Part model, mm, in its own coordinate system. A direction names the side the tool comes from. Give positions to 0.01 mm unless a question says otherwise; leave off trailing zeros. Write each loop counter-clockwise with the first axis right and the second up, starting at its lowest first coordinate (ties: lowest second). Pieces come first, ordered by that corner, then holes.
Autodesk Fusion 360 part; units mm, degrees
sketch "Sketch1" plane through (0, 0, 0) normal (0, 0, 1) x (1, 0, 0)
  line L0 (0, 0) -> (-180, 0)
  line L1 (-180, 0) -> (-180, 105)
  line L2 (-180, 105) -> (0, 105)
  line L3 (0, 105) -> (0, 0)
  dimension "d1" = 180
  dimension "d2" = 105
extrude "Extrude1" add sketch "Sketch1" along normal blind 15
sketch "Sketch2" plane through (0, 0, 15) normal (0, 0, 1) x (-1, 0, 0)
  line L0 (0, -105) -> (180, -105)
  line L1 (180, -105) -> (180, 0)
  line L2 (180, 0) -> (0, 0)
  line L3 (0, 0) -> (0, -105)
  line L4 (90, 0) -> (73, 0)
  line L5 (90, 0) -> (107, 0)
  line L6 (107, 0) -> (107, -12)
  line L7 (107, -12) -> (104, -12)
  line L8 (104, -12) -> (104, -3)
  line L9 (73, 0) -> (73, -12)
  line L10 (73, -12) -> (76, -12)
  line L11 (76, -12) -> (76, -3)
  line L12 (76, -3) -> (104, -3)
  dimension "d6" = 17
  dimension "d7" = 17
  dimension "d14" = 3
  dimension "d15" = 9
  dimension "d26" = 12
  dimension "d27" = 3
extrude "Extrude3" add sketch "Sketch2" along normal blind 115 contours L2 L4 L5 L6 L7 L8 L9 L10 L11 L12
sketch "Sketch4" plane through (0, 0, 130) normal (0, 0, 1) x (-1, 0, 0)
  line L0 (107, 0) -> (73, 0)
  line L1 (104, -3) -> (104, -12)
  line L2 (104, -12) -> (107, -12)
  line L3 (107, -12) -> (107, 0)
  line L4 (73, -12) -> (76, -12)
  line L5 (76, -12) -> (76, -3)
  line L6 (73, 0) -> (73, -12)
  line L7 (76, -3) -> (104, -3)
sketch "Sketch5" plane through (0, 0, 130) normal (0, 0, 1) x (-1, 0, 0)
  line L0 (76, -3) -> (104, -3)
  line L1 (104, -3) -> (104, -12)
  line L2 (104, -12) -> (76, -12)
  line L3 (76, -12) -> (76, -3)
  line L4 (76, -3) -> (104, -12)
  line L5 (76, -12) -> (104, -3)
  circle A0 centre (90, -7.5) radius 2
  dimension "d28" = 4
extrude "Extrude4" add sketch "Sketch5" against normal blind 3 contours L3 L4 L5 A0 | L0 L4 L5 A0 | L1 L4 L5 A0 | L2 L4 L5 A0
mirror "Mirror2" about plane through (-90, 52.5, 65) normal (0, -1, 0) of "Extrude3", "Extrude4"
ref_plane "WorkPlane3" through (-90, 52.5, 65) normal (0, 1, 0) x (-1, 0, 0)
fillet "Fillet2" radius 5 10 edges at (0, 52.5, 15) (0, 0, 7.5) (0, 105, 7.5) (-180, 52.5, 15) (-180, 105, 7.5) (-180, 0, 7.5) (-143.5, 0, 15) (-143.5, 105, 15) (-36.5, 0, 15) (-36.5, 105, 15)
1) Flat gauge pins, fed straight in: P1, Ø3.5, axis at y = 7, z = 57, coming from the -X side; P2, Ø6, axis at x = -155.5, z = 14, coming from the -Y side; P3, Ø3, axis at x = -47, z = 14.5, coming from the +Y side. Where does each tip first touch, or does it go through?
Check result:
P1: stops at x = -107
P2: stops at y = 0.1
P3: stops at y = 104
2) Saw through at B-B (x = -90). Write the cut outline in (y, z), and give its area (4 significant figures).
Check result:
outline: (0, 0) - (105, 0) - (105, 130) - (99.5, 130) - (99.5, 127) - (102, 127) - (102, 15) - (3, 15) - (3, 127) - (5.5, 127) - (5.5, 130) - (0, 130) - close; (9.5, 127) - (12, 127) - (12, 130) - (9.5, 130) - close; (93, 127) - (95.5, 127) - (95.5, 130) - (93, 130) - close
area: 2,295 mm2
3) Saw through at D-D (y = 7.5). Write the cut outline in (x, z).
Check result:
outline: (-180, 0) - (0, 0) - (0, 10) arc R5 ccw to (-5, 15) - (-73, 15) - (-73, 130) - (-88, 130) - (-88, 127) - (-76, 127) - (-76, 15) - (-104, 15) - (-104, 127) - (-92, 127) - (-92, 130) - (-107, 130) - (-107, 15) - (-175, 15) arc R5 ccw to (-180, 10) - close
4) 3-axis set-ups, long thin cutter, end or side, ignore diameter. For faces 4 (the flat face through (-90, 100, 127)), 5 (the cylindrical face through (-91.908, 6.899, 128.521)), 6 (the cylindrical face through (-39, 1, 13)): which of +Z, -Z, +X, -X, +Y, -Y reach the whole face in a straight line?
Check result:
face 4: none
face 5: +Z
face 6: +Z, +X, -Y
5) Saw through at A-A (z = 20.5). Write the cut outline in (x, y).
Check result:
outline: (-107, 0) - (-73, 0) - (-73, 12) - (-76, 12) - (-76, 3) - (-104, 3) - (-104, 12) - (-107, 12) - close; (-107, 93) - (-104, 93) - (-104, 102) - (-76, 102) - (-76, 93) - (-73, 93) - (-73, 105) - (-107, 105) - close
6) Drill centre lines: L1, parallel to Y at x = -90, z = 128.65; L2, parallel to Y at x = -99, z = 29.5; L3, parallel to Z at x = -148, y = 77.5. Where is each one in solid material? Low to high.
Check result:
L1: y = 0 to 5.5, 9.5 to 12, 93 to 95.5, 99.5 to 105
L2: y = 0 to 3, 102 to 105
L3: z = 0 to 15
7) Saw through at C-C (x = -130.5). Write the cut outline in (y, z).
Check result:
outline: (0, 0) - (105, 0) - (105, 10) arc R5 ccw to (100, 15) - (5, 15) arc R5 ccw to (0, 10) - close
8) Mould opens along X. For faces 1 (the cylindrical face through (-179, 2, 5)), 2 (the flat face through (-76, 8, 70)), 3 (the cylindrical face through (-1, 103, 5)) say: +X half, -X half, draft (parallel to the pull), parting line (faces both ways), or undercut.
Check result:
face 1: -X half
face 2: undercut
face 3: +X half
